from build123d import *

# Parameters (mm, degrees)
SKIZZE2_R              = 72.5
BASE_DEPTH             = 32
SKIZZE3_W              = 1
SKIZZE3_H              = 0.5
SKIZZE4_W              = 28
SKIZZE4_H              = 38
FRONT_CAMERA_CUT_DEPTH = 17.5
SKIZZE5_W              = 1
SKIZZE5_H              = 38
FRONT_DETAIL_DEPTH     = 1
SKIZZE6_R              = 3.5
CAMERA_DETAIL_DEPTH    = 1


with BuildPart() as part:
    # Skizze2 → Base (new body)
    with BuildSketch(Plane.XY):
        Circle(SKIZZE2_R)
    extrude(amount=BASE_DEPTH)

    # Skizze3 → Cover Seam (revolve, cut)
    with BuildSketch(Plane(origin=(0, 0, 0), x_dir=(1, 0, 0), z_dir=(0, 1, 0)), mode=Mode.PRIVATE) as cover_seam_sk:
        with Locations((72, -2.25)):
            Rectangle(SKIZZE3_W, SKIZZE3_H)
    revolve(cover_seam_sk.sketch.rotate(Axis((0, 0, 0), (0, 0, 1)), 180), axis=Axis((0, 0, 0), (0, 0, 1)), mode=Mode.SUBTRACT)

    # Skizze4 → Front Camera Cut (cut)
    with BuildSketch(Plane(origin=(72.5, 0, 0), x_dir=(0, 0, -1), z_dir=(1, 0, 0))):
        with Locations((-16, 0)):
            Rectangle(SKIZZE4_W, SKIZZE4_H)
    extrude(amount=-FRONT_CAMERA_CUT_DEPTH, mode=Mode.SUBTRACT)

    # Skizze5 → Front Detail (cut)
    with BuildSketch(Plane(origin=(55, 0, 0), x_dir=(0, 0, -1), z_dir=(1, 0, 0))):
        with Locations((-29.5, 0)):
            Rectangle(SKIZZE5_W, SKIZZE5_H)
    extrude(amount=-FRONT_DETAIL_DEPTH, mode=Mode.SUBTRACT)

    # Skizze6 → Camera Detail (add)
    with BuildSketch(Plane(origin=(55, 0, 0), x_dir=(0, 0, -1), z_dir=(1, 0, 0))):
        with Locations(Location((-16, 0, 0), (0, 0, 180))):
            Circle(SKIZZE6_R)
    extrude(amount=CAMERA_DETAIL_DEPTH)


solid = part.part
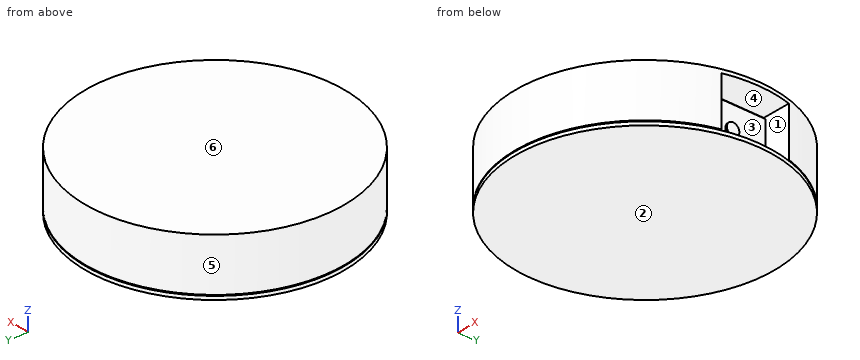
Can you work these out from the model? Positions are in its coordinate system, mm. Face numbers are marked on the shaded views. A direction names the side the tool comes from. Coordinates: 2 decimals unless noted, no trailing zeros. Write each loop counter-clockwise with the first axis right and the second up, starting at its lowest first coordinate (ties: lowest second). Pieces come first, ordered by that corner, then holes. Notation, with made-up numbers: (52, 37) -> (63, 37) arc R9 ccw to (63, 49) -> close; hole circle Ø4 at (58.25, 75). An arc over 180 degrees is marked (long way). Write each question's results on one line, items separated by ' | '. Start each with the question number.
Item 1: If we section it at A-A, the plane y = 0: Write out the boundary of the cut face in (x, z), and give its area (3 significant figures).
Item 2: Please list where these lines run through material, in increasing order: probe 1 along Y at (x, z) = (12, 21); probe 2 along Y at (x, z) = (65.5, 18.5); probe 3 along Y at (x, z) = (28, 11.5).
Item 3: Thinking about a two-plate mould opening in Y: for the marked faces 3, 4, 5 and 6, which applies, released by +Y, released by -Y, zero draft, split by the parting line, or undercut?
Item 4: I'm going to push flat-ended pins straight in: P1, Ø5.5, axis at y = 0, z = 16, coming from the +X side; P2, Ø3, axis at x = 25.5, z = 11, coming from the -Y side; P3, Ø2, axis at x = -31, z = 5, coming from the -Y side. Where does each tip first touch, or does it pass through?
Item 5: On a 3-axis mill with a long thin cutter (end or side, diameter ignored), from which of +Z, -Z, +X, -X, +Y, -Y can I reach the whole of each face in a straight line? I mean the marked faces 1 and 2. Say none if no direction works.
Item 6: If we section it at B-B, the plane z = 16: Write out the boundary of the cut face in (x, y), and give its area (3 significant figures).
Item 7: If we section it at D-D, the plane x = 47: Write out the boundary of the cut face in (y, z), and give its area (3 significant figures).
Item 8: If we section it at C-C, the plane x = -64: Write out the boundary of the cut face in (y, z), and give its area (3 significant figures).
Answer block:
1) outline: (-72.5, 0) -> (72.5, 0) -> (72.5, 2) -> (55, 2) -> (55, 12.5) -> (56, 12.5) -> (56, 19.5) -> (55, 19.5) -> (55, 29) -> (54, 29) -> (54, 30) -> (72.5, 30) -> (72.5, 32) -> (-72.5, 32) -> (-72.5, 2.5) -> (-71.5, 2.5) -> (-71.5, 2) -> (-72.5, 2) -> close | area: 4,160 mm²
2) probe 1: -71.5 to 71.5 | probe 2: -31.08 to -19, 19 to 31.08 | probe 3: -66.87 to 66.87
3) face 3: undercut | face 4: undercut | face 5: split by the parting line | face 6: zero draft
4) P1: x = 56 | P2: y = -68.41 | P3: y = -66
5) face 1: +X | face 2: -Z, +X, -X, +Y, -Y
6) outline: (55, -19) -> (55, -3.5) -> (56, -3.5) -> (56, 3.5) -> (55, 3.5) -> (55, 19) -> (69.97, 19) arc R72.5 ccw (long way) to (69.97, -19) -> close | area: 15,900 mm²
7) outline: (-55.2, 0) -> (55.2, 0) -> (55.2, 2) -> (53.88, 2) -> (53.88, 2.5) -> (55.2, 2.5) -> (55.2, 32) -> (-55.2, 32) -> (-55.2, 2.5) -> (-53.88, 2.5) -> (-53.88, 2) -> (-55.2, 2) -> close | area: 3,530 mm²
8) outline: (-34.06, 0) -> (34.06, 0) -> (34.06, 2) -> (31.88, 2) -> (31.88, 2.5) -> (34.06, 2.5) -> (34.06, 32) -> (-34.06, 32) -> (-34.06, 2.5) -> (-31.88, 2.5) -> (-31.88, 2) -> (-34.06, 2) -> close | area: 2,180 mm²
